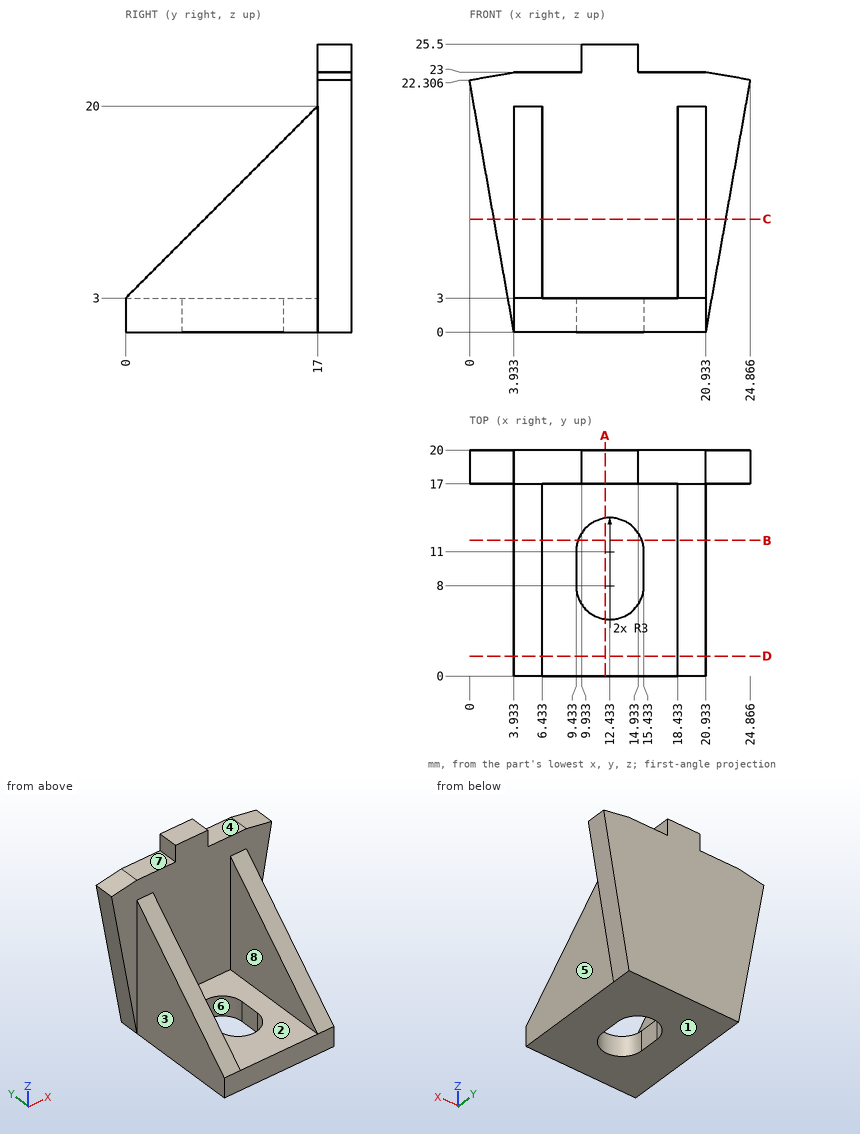
Source: three-view drawing plus pictorial views. Frame: mm from the lowest corner of the part. A direction names the side the tool comes from. Give positions to 0.01 mm unless a question says otherwise; leave off trailing zeros. Loops run counter-clockwise (first coordinate to the right, second up) from the corner with the lowest first, then second, coordinate; pieces in that order, holes last.
1) Line query: L1, parallel to X at y = 8.5, z = 4; L2, parallel to X at y = 11, z = 2.75; L3, parallel to Y at x = 10.75, z = 7.5. Output: solid intervals per line, ascending.
A:
L1: x = 3.93 to 6.43, 18.43 to 20.93
L2: x = 3.93 to 9.43, 15.43 to 20.93
L3: y = 17 to 20
2) Section query C-C on z = 10. Return the cut outline in (x, y).
A:
outline: (2.17, 17) - (3.93, 17) - (3.93, 7) - (6.43, 7) - (6.43, 17) - (18.43, 17) - (18.43, 7) - (20.93, 7) - (20.93, 17) - (22.7, 17) - (22.7, 20) - (2.17, 20) - close
3) Contact query for flat-ended pins moving along their axis: pin 1 (1.5 mm diameter, centred on y = 10, z = 1, fed in from +X); pin 2 (8 mm diameter, centred on x = 5, y = 3, fed in from +Z); pin 3 (0.8 mm diameter, centred on y = 18, z = 24.5, fed in from -X). Output: stop coordinate, or through.
A:
pin 1: stops at x = 20.93
pin 2: stops at z = 10
pin 3: stops at x = 9.93
4) Section query B-B on y = 12. Return the cut outline in (x, z) (1 decimal).
A:
outline: (3.9, 0) - (9.6, 0) - (9.6, 3) - (6.4, 3) - (6.4, 15) - (3.9, 15) - close; (15.3, 0) - (20.9, 0) - (20.9, 15) - (18.4, 15) - (18.4, 3) - (15.3, 3) - close
5) Section query D-D on y = 1.75. Return the cut outline in (x, z).
A:
outline: (3.93, 0) - (20.93, 0) - (20.93, 4.75) - (18.43, 4.75) - (18.43, 3) - (6.43, 3) - (6.43, 4.75) - (3.93, 4.75) - close
6) Mould query, pull axis X, two halves, no side actions, for the marked faces 1, 2 and 3. Classes: released by +X, released by -X, zero draft, split by the parting line, or undercut.
A:
face 1: zero draft
face 2: undercut
face 3: released by -X
7) Section query A-A on x = 12. Return the cut outline in (y, z), and give its area (3 significant figures).
A:
outline: (0, 0) - (5.03, 0) - (5.03, 3) - (0, 3) - close; (13.97, 0) - (20, 0) - (20, 25.5) - (17, 25.5) - (17, 3) - (13.97, 3) - close
area: 101 mm2
8) Reachability of the marked faces 4, 5, 6, 7 and 8 from +Z, -Z, +X, -X, +Y, -Y: full face, straight path, thin tool, end or side. Return the list, or none.
A:
face 4: +Z, +X, +Y, -Y
face 5: +Z, -Z, +X, -Y
face 6: +Z, -Z
face 7: +Z, -X, +Y, -Y
face 8: +Z, -Y
